Could you check a few things on this model? Use its own coordinates, in mm. Face numbers are marked on the shaded views. A direction names the side the tool comes from. Round coordinates to 2 decimals unless told otherwise and drop trailing zeros. Write each loop counter-clockwise with the first axis right and the second up, starting at its lowest first coordinate (ties: lowest second). Pieces come first, ordered by that corner, then holes. Notation, with made-up numbers: M 8.25,-2.75 L 56.25,-2.75 A17 cw 56.25,25.25 Z; hole C 13,73.25 d6. An arc over 180 degrees is marked long. One line per question, with ' | ' between items. Start each with the question number.
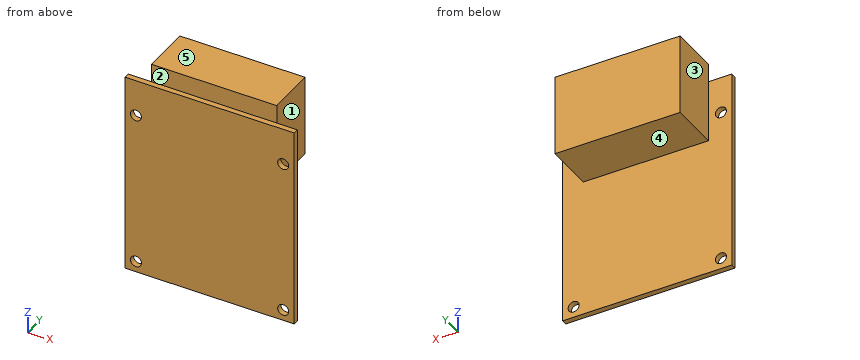
Autodesk Inventor part; units mm, degrees
ref_plane "YZ Plane" through (0, 0, 0) normal (1, 0, 0) x (0, 1, 0)
ref_plane "XZ Plane" through (0, 0, 0) normal (0, 1, 0) x (-1, 0, 0)
ref_plane "XY Plane" through (0, 0, 0) normal (0, 0, 1) x (1, 0, 0)
sketch "Sketch1" plane through (0, 0, 0) normal (0, 1, 0) x (-1, 0, 0)
  line L0 (-23, 27.5) -> (23, 27.5)
  line L1 (23, 27.5) -> (23, -27.5)
  line L2 (23, -27.5) -> (-23, -27.5)
  line L3 (-23, -27.5) -> (-23, 27.5)
  line L4 (-23, 27.5) -> (23, -27.5) construction
  line L5 (23, 27.5) -> (-23, -27.5) construction
  point P0 (0, 0)
  dimension "d0" = 46
  dimension "d1" = 55
extrude "Extrusion1" add sketch "Sketch1" along normal blind 1.5
sketch "Sketch2" plane through (0, 1.5, 0) normal (0, 1, 0) x (1, 0, 0)
  line L0 (-16.6, -32.5) -> (17.4, -32.5)
  line L1 (17.4, -32.5) -> (17.4, -10.5)
  line L2 (17.4, -10.5) -> (-16.6, -10.5)
  line L3 (-16.6, -10.5) -> (-16.6, -32.5)
  line L4 (-16.6, -32.5) -> (17.4, -10.5) construction
  line L5 (17.4, -32.5) -> (-16.6, -10.5) construction
  line L6 (-23, -27.5) -> (23, -27.5)
  line L7 (-23, 27.5) -> (-23, -27.5)
  point P0 (0, 0)
  point P1 (0.4, -21.5)
  dimension "d4" = 34
  dimension "d5" = 22
  dimension "d6" = 5
  dimension "d7" = 6.4
extrude "Extrusion2" add sketch "Sketch2" along normal blind 13.4
sketch "Sketch3" plane through (0, 0, 0) normal (0, -1, 0) x (1, 0, 0)
  line L0 (20, 17.5) -> (-20, 17.5) construction
  line L1 (-20, 17.5) -> (-20, -24.5) construction
  line L2 (-20, -24.5) -> (20, -24.5) construction
  line L3 (20, -24.5) -> (20, 17.5) construction
  line L4 (23, -27.5) -> (23, 27.5) construction
  line L5 (-23, 27.5) -> (-23, -27.5)
  line L6 (-23, -27.5) -> (23, -27.5)
  point P0 (0, 0)
  dimension "d10" = 42
  dimension "d11" = 40
  dimension "d12" = 3
  dimension "d13" = 3
  dimension "d14" = 3
hole "Hole1" at (20, 0, 17.5) at (-20, 0, 17.5) at (-20, 0, -24.5) at (20, 0, -24.5) direction (0, 1, 0) diameter 3 end through all
equation "\"d13\" = d12"
equation "\"d14\" = d12"
properties part number "board"
1. Suppose I cut it at D-D (y = 3.75). Write out the boundary of the cut face in (x, z), and give its area (3 significant figures).
2. Suppose I cut it at B-B (x = 20). Write out the boundary of the cut face in (y, z).
3. I need wall thicknesses on line 1 along Z through (x, y) = (-20, 1.05); line 2 along X through (y, z) = (0.3, 17.5); line 3 along Z through (x, y) = (-14.5, 5). Which ranges of each line are inside material? Lowest first, please. Write a range as from..to.
4. I'm going to push flat-ended pins straight in: P1, Ø1.8, axis at x = -20, z = -24.5, coming from the -Y side; P2, Ø6.5, axis at y = 11, z = 20.5, coming from the +X side; P3, Ø1.5, axis at y = 12.5, z = 16.5, coming from the -X side; P4, Ø1, axis at x = -15, z = -2, coming from the +Y side. Where does each tip first touch, or does it pass through?
5. Which directions (+Z, -Z, +X, -X, +Y, -Y) give clear straight access to the entire face, cutting with the end or side of a thin tool? Please do the marked faces 1, 2, 3, 4 and 5.
6. Suppose I cut it at C-C (z = -24.5). Write out the boundary of the cut face in (x, y).
7. Suppose I cut it at A-A (z = 17.5). Write out the boundary of the cut face in (x, y), and give its area (3 significant figures).
Computed:
1) outline: M -16.6,10.5 L 17.4,10.5 L 17.4,32.5 L -16.6,32.5 Z | area: 748 mm²
2) outline: M 0,-27.5 L 1.5,-27.5 L 1.5,-26 L 0,-26 Z; M 0,-23 L 1.5,-23 L 1.5,16 L 0,16 Z; M 0,19 L 1.5,19 L 1.5,27.5 L 0,27.5 Z
3) line 1: z = -27.5..-26, -23..16, 19..27.5 | line 2: x = -23..-21.5, -18.5..18.5, 21.5..23 | line 3: z = 10.5..32.5
4) P1: passes through | P2: stops at x = 17.4 | P3: stops at x = -16.6 | P4: stops at y = 1.5
5) face 1: +Z, -Z, +X, +Y | face 2: +Z, +X, -X, -Y | face 3: +Z, -Z, -X, +Y | face 4: -Z, +X, -X, +Y | face 5: +Z, +X, -X, +Y, -Y
6) outline: M -23,0 L -21.5,0 L -21.5,1.5 L -23,1.5 Z; M -18.5,0 L 18.5,0 L 18.5,1.5 L -18.5,1.5 Z; M 21.5,0 L 23,0 L 23,1.5 L 21.5,1.5 Z
7) outline: M -23,0 L -21.5,0 L -21.5,1.5 L -23,1.5 Z; M -18.5,0 L 18.5,0 L 18.5,1.5 L 17.4,1.5 L 17.4,14.9 L -16.6,14.9 L -16.6,1.5 L -18.5,1.5 Z; M 21.5,0 L 23,0 L 23,1.5 L 21.5,1.5 Z | area: 516 mm²
